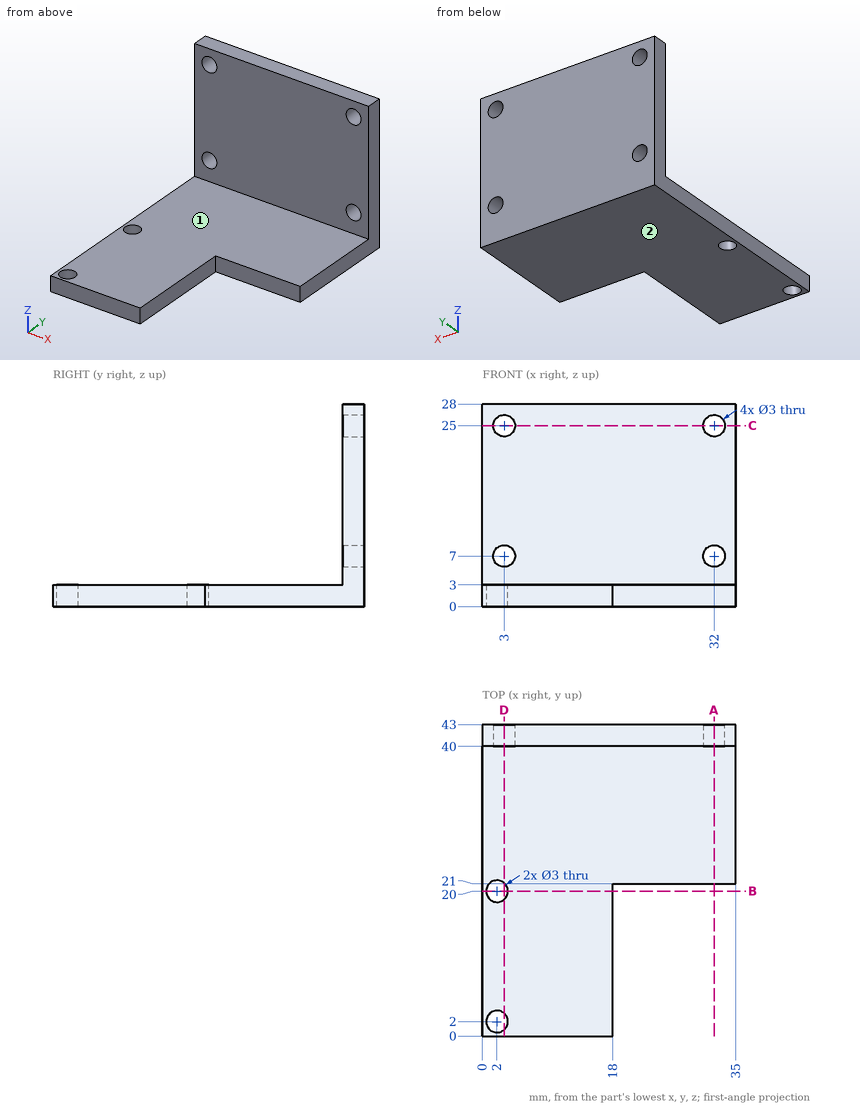
Source: three-view drawing plus pictorial views. Frame: mm from the lowest corner of the part. A direction names the side the tool comes from. Round coordinates to 2 decimals unless told otherwise and drop trailing zeros. Loops run counter-clockwise (first coordinate to the right, second up) from the corner with the lowest first, then second, coordinate; pieces in that order, holes last. Notation, with made-up numbers: M -28,88 L -18,88 A13 ccw -18,112 Z; hole C 78.25,-8.75 d5. An arc over 180 degrees is marked long. Answer as CSV lines item,"result".
Q1. Cut plane C-C (z = 25). Return the cut outline in (x, y).
Verdict:
outline,"M 0,40 L 1.5,40 L 1.5,43 L 0,43 Z; M 4.5,40 L 30.5,40 L 30.5,43 L 4.5,43 Z; M 33.5,40 L 35,40 L 35,43 L 33.5,43 Z"
Q2. Reachability of the marked faces 1 and 2 from +Z, -Z, +X, -X, +Y, -Y: full face, straight path, thin tool, end or side. Return the list, or none.
Verdict:
face 1,"+Z, +X, -X, -Y"
face 2,"-Z, +X, -X, +Y, -Y"
Q3. Cut plane B-B (y = 20). Return the cut outline in (x, z), plus the area to 3 significant figures.
Verdict:
outline,"M 0,0 L 0.5,0 L 0.5,3 L 0,3 Z; M 3.5,0 L 18,0 L 18,3 L 3.5,3 Z"
area,"45.0 mm^2"
Q4. Line query: line 1 along Y through (x, z) = (2, 1.35); line 2 along Z through (x, y) = (10.5, 15.5); line 3 along Y through (x, z) = (25, 20.75). Output: solid intervals per line, ascending.
Verdict:
line 1,"y = 0 to 0.5, 3.5 to 18.5, 21.5 to 43"
line 2,"z = 0 to 3"
line 3,"y = 40 to 43"
Q5. Cut plane D-D (x = 3). Return the cut outline in (y, z), plus the area to 3 significant figures.
Verdict:
outline,"M 0,0 L 0.88,0 L 0.88,3 L 0,3 Z; M 3.12,0 L 18.88,0 L 18.88,3 L 3.12,3 Z; M 21.12,0 L 43,0 L 43,5.5 L 40,5.5 L 40,3 L 21.12,3 Z; M 40,8.5 L 43,8.5 L 43,23.5 L 40,23.5 Z; M 40,26.5 L 43,26.5 L 43,28 L 40,28 Z"
area,"173 mm^2"
Q6. Contact query for flat-ended pins moving along their axis: pin 1 (3.5 mm diameter, centred on x = 32, z = 25, fed in from -Y); pin 2 (1 mm diameter, centred on x = 15, y = 27, fed in from +Z); pin 3 (0.9 mm diameter, centred on y = 11, z = 1, fed in from +X). Output: stop coordinate, or through.
Verdict:
pin 1,"stops at y = 40"
pin 2,"stops at z = 3"
pin 3,"stops at x = 18"
Q7. Cut plane A-A (x = 32). Return the cut outline in (y, z), plus the area to 3 significant figures.
Verdict:
outline,"M 21,0 L 43,0 L 43,5.5 L 40,5.5 L 40,3 L 21,3 Z; M 40,8.5 L 43,8.5 L 43,23.5 L 40,23.5 Z; M 40,26.5 L 43,26.5 L 43,28 L 40,28 Z"
area,"123 mm^2"
